Autodesk Inventor part; units mm, degrees
ref_plane "YZ Plane" through (0, 0, 0) normal (1, 0, 0) x (0, 1, 0)
ref_plane "XZ Plane" through (0, 0, 0) normal (0, 1, 0) x (-1, 0, 0)
ref_plane "XY Plane" through (0, 0, 0) normal (0, 0, 1) x (1, 0, 0)
sketch "Sketch1" plane through (0, 0, 0) normal (0, 1, 0) x (-1, 0, 0)
  circle A0 centre (0, 0) radius 1.5
  dimension "d0" = 3
extrude "Extrusion1" add sketch "Sketch1" along normal blind 40
sketch "Sketch2" plane through (0, 40, 0) normal (0, 1, 0) x (1, 0, 0)
  circle A0 centre (0, 0) radius 0.75
  dimension "d3" = 1.5
extrude "Extrusion2" cut sketch "Sketch2" against normal blind 40
chamfer "Chamfer1" distance 0.25 angle 45 2 edges at (1.5, 40, 0) (1.5, 0, 0)
properties part number "pin_3_40"
For this review, take the finished solid that the model builds, in its own axes (mm). Give positions to 0.01 mm unless a question says otherwise; leave off trailing zeros. Order: outer loops, then holes, each group sorted by start corner. A loop starts at its lowest first (then second) coordinate and runs counter-clockwise, first axis right, second up.
1) Take a section at B-B (z = 0). Give the boundary of the cut face in (x, y).
2) The part is to be moulded in two halves that separate along X. For faces 1 (the face through (-1, 40, 0)), 2 (the face through (-0.75, 20.28, -0.03)), 3 (the face through (1.5, 19.72, -0.07)), say which applies: released by +X, released by -X, zero draft, split by the parting line, or undercut.
3) Take a section at A-A (x = 0). Give the boundary of the cut face in (y, z), then the cut area to 3 significant figures.
4) Insertion check: pin 1 (1.5 mm diameter, centred on x = -1, y = 29.5, fed in from -Z). The pin has a flat end and moves straight along its axis. Give the tip position at first contact, or say it passes through.
5) Take a section at C-C (y = 13.5). Give the boundary of the cut face in (x, z), then the cut area to 3 significant figures.
6) Wall thickness on line 1 (Z direction, x = 0, y = 16); line 2 (X direction, y = 25.5, z = -0.1); line 3 (Y direction, x = 1.25, z = 0.05): over which ranges is each line inside the solid? List them lowest first.
Derived:
1. outline: (-1.5, 0.25) - (-1.25, 0) - (-0.75, 0) - (-0.75, 40) - (-1.25, 40) - (-1.5, 39.75) - close; (0.75, 0) - (1.25, 0) - (1.5, 0.25) - (1.5, 39.75) - (1.25, 40) - (0.75, 40) - close
2. face 1: zero draft
2. face 2: undercut
2. face 3: split by the parting line
3. outline: (0, -1.25) - (0.25, -1.5) - (39.75, -1.5) - (40, -1.25) - (40, -0.75) - (0, -0.75) - close; (0, 0.75) - (40, 0.75) - (40, 1.25) - (39.75, 1.5) - (0.25, 1.5) - (0, 1.25) - close
3. area: 59.9 mm2
4. pin 1: stops at z = -1.48
5. outline: circle Ø3 at (0, 0); hole circle Ø1.5 at (0, 0)
5. area: 5.30 mm2
6. line 1: z = -1.5 to -0.75, 0.75 to 1.5
6. line 2: x = -1.5 to -0.74, 0.74 to 1.5
6. line 3: y = 0 to 40
